The listing builds one solid part. Answer for the finished solid, in the listing's coordinates (mm). A direction names the side the tool comes from. Round coordinates to 2 decimals unless told otherwise and drop trailing zeros. Order: outer loops, then holes, each group sorted by start corner. A loop starts at its lowest first (then second) coordinate and runs counter-clockwise, first axis right, second up. Notation, with made-up numbers: (53, -16.5) - (88, -16.5) arc R9 cw to (88, -6.5) - close; hole circle Ø10 at (21, 25.25). An arc over 180 degrees is marked (long way). Use CSV: the item, a comma, the result in double quotes. Start each with the question number.
Item 1: Find section D-D, the plane x = -13.75. Give the vertices of the cut face in (y, z), plus the area to 3 significant figures.
Item 2: Find section C-C, the plane x = -17.25. Give the vertices of the cut face in (y, z).
Item 3: Flat-ended cylindrical pins translate along their axes: P1, Ø1, axis at x = -10, z = -11, coming from the -Y side; P2, Ø8, axis at x = -17, y = 20.5, coming from the +Z side; P3, Ø4, axis at x = -16.5, y = 0, coming from the -Z side; P4, Ø1, axis at y = 21.5, z = -1, coming from the -X side. Find the tip coordinate at first contact, or state that the pin passes through.
Item 4: Straight lines are drawn through the part: line 1 along Z through (x, y) = (-0.9, 0); line 2 along X through (y, z) = (10, 25); line 3 along Z through (x, y) = (-14.25, 0). For each, find the intervals that lie inside material, in ascending order. Write a range as [from, to].
Item 5: For faces 4 (the cylindrical face through (-17.263, -5.961, -26.846)), 5 (the cylindrical face through (-9.004, -20.633, -15.821)), 6 (the flat face through (-3, -16, 25)), determine the directions among +Z, -Z, +X, -X, +Y, -Y from which every point of the face is accessible in a straight line to the end or side of a thin tool.
Item 6: Determine the mould class of faces 1 (the flat face through (-16.3, -10.1, -24.3)), 2 (the flat face through (-1.5, -8, -23)), 3 (the cylindrical face through (-0.76, -23.977, 1.055)) for opening direction X: +X half, -X half, draft (parallel to the pull), parting line (faces both ways), or undercut.
Item 7: Find section A-A, the plane z = 0. Give the vertices of the cut face in (x, y).
```python
from build123d import *

# Parameters (mm, degrees)
CHAMFER_1_SIZE = 0.5


with BuildPart() as part:
    # Эскиз1 → Повернуть1 (revolve)
    with BuildSketch(Plane.XY):
        Polygon((0, 24), (-1.5, 24), (-1.5, 26), (-16.3, 26), (-16.3, 27.5), (-18.2, 27.5), (-18.2, 26), (-19.7, 26), (-19.7, 30), (-3, 30), (-3, 29), (0, 29), align=None)
    revolve(axis=Axis((-1000, 0, 0), (1, 0, 0)))

    # Фаска1
    chamfer_1_edges = [part.edges().sort_by_distance(p)[0] for p in [
        (-19.7, -30, 0),
    ]]
    chamfer(chamfer_1_edges, length=CHAMFER_1_SIZE)


solid = part.part
```
Worked out:
1,outline,"circle Ø60 at (0, 0); hole circle Ø52 at (0, 0)"
1,area,"704 mm²"
2,outline,"circle Ø60 at (0, 0); hole circle Ø55 at (0, 0)"
3,P1,"stops at y = -28.1"
3,P2,"stops at z = 25.05"
3,P3,"stops at z = -30"
3,P4,"passes through"
4,line 1,"z = [-29, -24], [24, 29]"
4,line 2,"x = [-19.7, -18.2], [-16.3, 0]"
4,line 3,"z = [-30, -26], [26, 30]"
5,face 4,"none"
5,face 5,"-X"
5,face 6,"+X"
6,face 1,"undercut"
6,face 2,"-X half"
6,face 3,"draft"
7,outline,"(-19.7, -29.5) - (-19.2, -30) - (-3, -30) - (-3, -29) - (0, -29) - (0, -24) - (-1.5, -24) - (-1.5, -26) - (-16.3, -26) - (-16.3, -27.5) - (-18.2, -27.5) - (-18.2, -26) - (-19.7, -26) - close; (-19.7, 26) - (-18.2, 26) - (-18.2, 27.5) - (-16.3, 27.5) - (-16.3, 26) - (-1.5, 26) - (-1.5, 24) - (0, 24) - (0, 29) - (-3, 29) - (-3, 30) - (-19.2, 30) - (-19.7, 29.5) - close"
